Solid Edge part; units mm, degrees
sketch "Sketch1" plane through (0, 0, 0) normal (1, 0, 0) x (0, 1, 0)
  line L0 (0, 0) -> (43.8289, 0)
sketch "Sketch2" plane through (0, 0, 0) normal (0, -1, 0) x (1, 0, 0)
  line L0 (0, 101.6) -> (0, 0)
  line L1 (0, 0) -> (6.35, 0)
  line L2 (6.35, 44.45) -> (6.35, 0)
  line L3 (50.8, 44.45) -> (6.35, 44.45)
  line L4 (50.8, 50.8) -> (50.8, 44.45)
  line L5 (6.35, 50.8) -> (50.8, 50.8)
  line L6 (6.35, 95.25) -> (6.35, 50.8)
  line L7 (6.35, 95.25) -> (50.8, 95.25)
  line L8 (50.8, 95.25) -> (50.8, 101.6)
  line L9 (50.8, 101.6) -> (0, 101.6)
sweep "SweptProtrusion_1" add profiles "Sketch2" path "Sketch1"
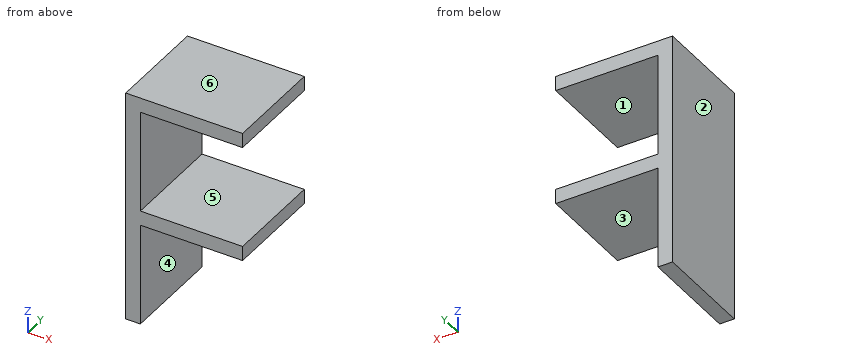
Work out the finished part from the listing and answer in its coordinate system (mm). Face numbers are marked on the shaded views. A direction names the side the tool comes from. Give positions to 0.01 mm unless a question says otherwise; leave off trailing zeros. Order: outer loops, then holes, each group sorted by start corner. A loop starts at its lowest first (then second) coordinate and runs counter-clockwise, first axis right, second up. Notation, with made-up numbers: (89, -36) -> (95, -36) arc R31 cw to (95, -11) -> close; hole circle Ø6 at (-13, 36.5). An arc over 180 degrees is marked (long way). Answer as CSV lines item,"result". Start each with the question number.
(1) Section B-B, the plane y = 9.5 is taken. Write down the section's boundary in (x, z).
(2) Each of these flat-tipped pins is pushed along its axis until it touches: pin 1 Ø2 at (y, z) = (26, 52) entering from +X; pin 2 Ø2 at (x, y) = (24.5, 22.5) entering from -Z. Where does it stop, or does it pass through?
(3) Which of the six approach directions +Z, -Z, +X, -X, +Y, -Y give full straight-line access (tool end or side, diameter ignored) to the marked faces 4, 5 and 6?
(4) Section C-C, the plane z = 28 is taken. Write down the section's boundary in (x, y).
(5) For a pull along Z with two mould halves and no side action, classify the marked faces 1, 2 and 3 as released by +Z, released by -Z, zero draft, split by the parting line, or undercut.
(6) Consider line 1 along Z through (x, y) = (11, 29.5); line 2 along X through (y, z) = (32.5, 83.5). Determine where each line is inside the solid, lowest interval first.
(7) Section A-A, the plane x = 21 is taken. Write down the section's boundary in (y, z).
Entries:
1,outline,"(0, 0) -> (6.35, 0) -> (6.35, 44.45) -> (50.8, 44.45) -> (50.8, 50.8) -> (6.35, 50.8) -> (6.35, 95.25) -> (50.8, 95.25) -> (50.8, 101.6) -> (0, 101.6) -> close"
2,pin 1,"x = 6.35"
2,pin 2,"z = 44.45"
3,face 4,"-Z, +X, +Y, -Y"
3,face 5,"+X, +Y, -Y"
3,face 6,"+Z, +X, -X, +Y, -Y"
4,outline,"(0, 0) -> (6.35, 0) -> (6.35, 43.83) -> (0, 43.83) -> close"
5,face 1,"undercut"
5,face 2,"zero draft"
5,face 3,"released by -Z"
6,line 1,"44.45 to 50.8, 95.25 to 101.6"
6,line 2,"0 to 6.35"
7,outline,"(0, 44.45) -> (43.83, 44.45) -> (43.83, 50.8) -> (0, 50.8) -> close; (0, 95.25) -> (43.83, 95.25) -> (43.83, 101.6) -> (0, 101.6) -> close"
